```python
from build123d import *

# Parameters (mm, degrees)
SKETCH_W        = 76
SKETCH_H        = 40
PAD_DEPTH       = 30
SKETCH001_W     = 44
SKETCH001_H     = 43.078728
POCKET_DEPTH    = 26
SKETCH002_R     = 2.3
POCKET001_DEPTH = 30.001
SKETCH003_W     = 14
SKETCH003_H     = 44.554736
SKETCH003_H_2   = 44
POCKET002_DEPTH = 26
POCKET003_DEPTH = 26
SKETCH005_R     = 11.5
SKETCH005_R_2   = 1.7
POCKET004_DEPTH = 5
FILLET_R        = 3


with BuildPart() as part:
    # Sketch → Pad (new body)
    with BuildSketch(Plane.XY):
        with Locations((0, 20)):
            Rectangle(SKETCH_W, SKETCH_H)
    extrude(amount=PAD_DEPTH)

    # Sketch001 → Pocket (cut)
    with BuildSketch(Plane.XY.offset(30)):
        with Locations((0, 23.539364)):
            Rectangle(SKETCH001_W, SKETCH001_H)
    extrude(amount=-POCKET_DEPTH, mode=Mode.SUBTRACT)

    # Sketch002 → Pocket001 (cut, through all)
    with BuildSketch(Plane.XY.offset(30)):
        with Locations((-32, 10)):
            Circle(SKETCH002_R)
        with Locations((-32, 30)):
            Circle(SKETCH002_R)
        with Locations((32, 10)):
            Circle(SKETCH002_R)
    extrude(amount=-POCKET001_DEPTH, mode=Mode.SUBTRACT)

    # Sketch003 → Pocket002 (cut)
    with BuildSketch(Plane(origin=(0, 0, 0), x_dir=(1, 0, 0), z_dir=(0, 0, -1))):
        with Locations((-33, -19.722632)):
            Rectangle(SKETCH003_W, SKETCH003_H)
        with Locations((33, -20)):
            Rectangle(SKETCH003_W, SKETCH003_H_2)
    extrude(amount=-POCKET002_DEPTH, mode=Mode.SUBTRACT)

    # Sketch004 → Pocket003 (cut)
    with BuildSketch(Plane.XY.offset(30)):
        Polygon((20, 42), (40, 42), (40, 16), (26, 16), (20, 10), align=None)
    extrude(amount=-POCKET003_DEPTH, mode=Mode.SUBTRACT)

    # Sketch005 → Pocket004 (cut)
    with BuildSketch(Plane(origin=(0, 0, 0), x_dir=(1, 0, 0), z_dir=(0, 0, -1))):
        with Locations((0, -22)):
            Circle(SKETCH005_R)
        with Locations((-15.5, -5.437484)):
            Circle(SKETCH005_R_2)
        with Locations((15.5, -5.437484)):
            Circle(SKETCH005_R_2)
        with Locations((15.5, -36.437484)):
            Circle(SKETCH005_R_2)
        with Locations((-15.5, -36.437484)):
            Circle(SKETCH005_R_2)
    extrude(amount=-POCKET004_DEPTH, mode=Mode.SUBTRACT)

    # Fillet
    fillet_edges = [part.edges().sort_by_distance(p)[0] for p in [
        (26, 40, 2),
        (38, 16, 28),
        (38, 0, 28),
        (-38, 40, 28),
        (-38, 0, 28),
    ]]
    fillet(fillet_edges, radius=FILLET_R)


solid = part.part
```
Source: CAD feature listing. Evaluate the final solid. Frame: model axes, mm. A direction names the side the tool comes from. Coordinates: 2 decimals unless noted, no trailing zeros. Write each loop counter-clockwise with the first axis right and the second up, starting at its lowest first coordinate (ties: lowest second). Pieces come first, ordered by that corner, then holes. Notation, with made-up numbers: (20.5, 18.5) -> (64.5, 18.5) arc R22 ccw to (64.5, 56.5) -> close; hole circle Ø6 at (-40, -19.75). An arc over 180 degrees is marked (long way). Return JSON: item names as keys, results as strings. Group by question number.
1) Section query A-A, the plane y = 22. Return loops of the section in (x, z), plus the area to 3 significant figures.
2) Mould query, pull axis Y, two halves, no side actions, for faces 6 (the face through (8, 13, 4)), 7 (the face through (-1.5, 10.6, 2)), 8 (the face through (31, 16, 28)). Classes: +Y half, -Y half, draft (parallel to the pull), parting line (faces both ways), or undercut.
3) Section query B-B, the plane z = 27. Return loops of the section in (x, y), plus the area to 3 significant figures.
4) Contact query for flat-ended pins moving along their axis: P1, Ø3, axis at x = -18.5, y = 35, coming from the +Z side; P2, Ø8, axis at y = 18, z = 19.5, coming from the +X side; P3, Ø5, axis at y = 8.5, z = 21.5, coming from the -X side. Output: stop coordinate, or through.
5) Set-up query: faces 1 (the face through (0, 2, 17)), 2 (the face through (-32, 20, 26)), 3 (the face through (16.28, 37.95, 1.97)), 4 (the face through (-37.14, 39.1, 28.03)), 5 (the face through (26, 11, 13)). Return all of +Z, -Z, +X, -X, +Y, -Y with unobstructed straight access to the full face (end or side cutting, diameter ignored); none if empty.
6) Section query C-C, the plane x = 15.5. Return loops of the section in (y, z).
7) Section query D-D, the plane x = 0. Return loops of the section in (y, z).
8) Ray query, line 1 along Y through (x, z) = (15.5, 1.75); line 2 along Y through (x, z) = (0, 2.2); line 3 along X through (y, z) = (13, 26.75). Return the intervals inside material, ascending.
From the geometry:
{
 "1": {"outline": "(-38, 26) -> (-26, 26) -> (-26, 0) -> (-11.5, 0) -> (-11.5, 4) -> (-22, 4) -> (-22, 30) -> (-38, 30) -> close; (11.5, 0) -> (26, 0) -> (26, 4) -> (11.5, 4) -> close", "area": "268 mm²"},
 "2": {"face 6": "draft", "face 7": "undercut", "face 8": "+Y half"},
 "3": {"outline": "(-38, 3) arc R3 ccw to (-35, 0) -> (35, 0) arc R3 ccw to (38, 3) -> (38, 13) arc R3 ccw to (35, 16) -> (26, 16) -> (22, 12) -> (22, 2) -> (-22, 2) -> (-22, 40) -> (-35, 40) arc R3 ccw to (-38, 37) -> close; hole circle Ø4.6 at (-32, 10); hole circle Ø4.6 at (-32, 30); hole circle Ø4.6 at (32, 10)", "area": "918 mm²"},
 "4": {"P1": "z = 4", "P2": "x = 26", "P3": "x = -26"},
 "5": {"face 1": "+Z, +Y", "face 2": "-Z, -X, +Y, -Y", "face 3": "+Z, -Z", "face 4": "+Z, -Z, -X, +Y", "face 5": "-Z, +X, +Y, -Y"},
 "6": {"outline": "(0, 0) -> (3.74, 0) -> (3.74, 4) -> (2, 4) -> (2, 30) -> (0, 30) -> close; (7.14, 0) -> (34.74, 0) -> (34.74, 4) -> (7.14, 4) -> close; (38.14, 0) -> (40, 0) -> (40, 4) -> (38.14, 4) -> close"},
 "7": {"outline": "(0, 0) -> (10.5, 0) -> (10.5, 4) -> (2, 4) -> (2, 30) -> (0, 30) -> close; (33.5, 0) -> (40, 0) -> (40, 4) -> (33.5, 4) -> close"},
 "8": {"line 1": "0 to 3.74, 7.14 to 34.74, 38.14 to 40", "line 2": "0 to 10.5, 33.5 to 40", "line 3": "-38 to -22, 23 to 38"}
}
